Here's how the part is built. I have some questions about the finished solid (model axes, mm). A direction names the side the tool comes from. Coordinates: 2 decimals unless noted, no trailing zeros. Loops run counter-clockwise (first coordinate to the right, second up) from the corner with the lowest first, then second, coordinate; pieces in that order, holes last. Notation, with made-up numbers: (-9.75, 67) -> (5.25, 67) arc R24 cw to (5.25, 78) -> close; hole circle Ø3 at (4, 65). An arc over 180 degrees is marked (long way). Answer as a JSON object with one key per item and string values. Group by question number.
1) Which directions (+Z, -Z, +X, -X, +Y, -Y) give clear straight access to the entire face, cutting with the end or side of a thin tool? Please do faces 1 (the flat face through (5, 0, 21)), 2 (the flat face through (0, -151, 0)).
2) I'm going to push flat-ended pins straight in: pin 1 (4 mm diameter, centred on y = 18.5, z = -7, fed in from +X); pin 2 (1 mm diameter, centred on x = 15, y = -120.5, fed in from +Z); pin 3 (12 mm diameter, centred on y = -0.5, z = 0, fed in from +X); pin 4 (6 mm diameter, centred on x = -17.5, y = 46.5, fed in from -Z). Where does each tip first touch, or does it pass through?
3) I need wall thicknesses on probe 1 along Y at (x, z) = (-13, 17); probe 2 along Y at (x, z) = (-17, 3.5); probe 3 along X at (y, z) = (71.5, -7). Which ranges of each line are inside material? Lowest first, please. Write a range as [from, to].
4) I want a section at A-A (y = -125). Write out the boundary of the cut face in (x, z), then the cut area to 3 significant figures.
5) I want a section at B-B (y = 50). Write out the boundary of the cut face in (x, z), then the cut area to 3 significant figures.
```python
from build123d import *

# Parameters (mm, degrees)
F0_R     = 19
F1_DEPTH = 151
F2_R     = 25
F3_DEPTH = 96.5
F4_R     = 2


with BuildPart() as f1:
    # F0 (on Front) → F1 (new body)
    with BuildSketch(Plane.XZ):
        Circle(F0_R)
    extrude(amount=F1_DEPTH)

    # F2 (on Front) → F3 (join)
    with BuildSketch(Plane.XZ):
        with Locations((-0.022302, 0.055295)):
            Circle(F2_R)
    extrude(amount=-F3_DEPTH)

    # F4
    f4_edges = [f1.edges().sort_by_distance(p)[0] for p in [
        (-19, -151, 0),
        (19, -75.5, 0),
        (-19, 0, 0),
        (-25.022302, 0, 0.055295),
        (-25.022302, 96.5, 0.055295),
    ]]
    fillet(f4_edges, radius=F4_R)


solid = f1.part
```
Determined:
{
 "1": {"face 1": "-Y", "face 2": "+Z, -Z, +X, -X, -Y"},
 "2": {"pin 1": "x = 24.46", "pin 2": "z = 12.28", "pin 3": "x = 24.98", "pin 4": "z = -20.33"},
 "3": {"probe 1": "[0, 96.5]", "probe 2": "[-150.97, 96.5]", "probe 3": "[-24.01, 23.96]"},
 "4": {"outline": "circle Ø38 at (0, 0)", "area": "1,130 mm^2"},
 "5": {"outline": "circle Ø50 at (-0.02, 0.06)", "area": "1,960 mm^2"}
}
